```python
from build123d import *

# Parameters (mm, degrees)
SKETCH_R     = 8
SKETCH_W     = 8.42
SKETCH_H     = 2.25
PAD_DEPTH    = 1
SKETCH001_R  = 7
SKETCH001_W  = 8.42
SKETCH001_H  = 2.25
PAD001_DEPTH = 7
SKETCH002_R  = 7
SKETCH002_W  = 7.5
SKETCH002_H  = 1.5
PAD002_DEPTH = 1


with BuildPart() as part:
    # Sketch → Pad (new body)
    with BuildSketch(Plane.XY):
        Circle(SKETCH_R)
        Rectangle(SKETCH_W, SKETCH_H, mode=Mode.SUBTRACT)
    extrude(amount=PAD_DEPTH)

    # Sketch001 (on Face6 of Pad) → Pad001 (join)
    with BuildSketch(Plane(origin=(0, 0, 0), x_dir=(1, 0, 0), z_dir=(0, 0, -1))):
        Circle(SKETCH001_R)
        Rectangle(SKETCH001_W, SKETCH001_H, mode=Mode.SUBTRACT)
    extrude(amount=PAD001_DEPTH)

    # Sketch002 (on Face9 of Pad001) → Pad002 (join)
    with BuildSketch(Plane(origin=(0, 0, -7), x_dir=(1, 0, 0), z_dir=(0, 0, -1))):
        Circle(SKETCH002_R)
        Rectangle(SKETCH002_W, SKETCH002_H, mode=Mode.SUBTRACT)
    extrude(amount=PAD002_DEPTH)


solid = part.part
```
Can you work these out from the model? Positions are in its coordinate system, mm. A direction names the side the tool comes from. Coordinates: 2 decimals unless noted, no trailing zeros. Loops run counter-clockwise (first coordinate to the right, second up) from the corner with the lowest first, then second, coordinate; pieces in that order, holes last. Notation, with made-up numbers: (-9, 61.5) -> (12, 61.5) arc R20 cw to (12, 81.5) -> close; hole circle Ø9 at (71, 84). An arc over 180 degrees is marked (long way). Answer as a JSON object with one key per item and string values.
1) Imagine slicing it at C-C (x = 0). Please give me the cut outline in (y, z) (3 decimals).
Results:
{"outline": "(-8, 0) -> (-7, 0) -> (-7, -8) -> (-0.75, -8) -> (-0.75, -7) -> (-1.125, -7) -> (-1.125, 1) -> (-8, 1) -> close; (0.75, -8) -> (7, -8) -> (7, 0) -> (8, 0) -> (8, 1) -> (1.125, 1) -> (1.125, -7) -> (0.75, -7) -> close"}
2) Imagine slicing it at B-B (z = -5). Please give me the cut outline in (x, y) (3 decimals).
Results:
{"outline": "circle Ø14 at (0, 0); hole (-4.21, -1.125) -> (4.21, -1.125) -> (4.21, 1.125) -> (-4.21, 1.125) -> close"}
3) If I drill on line 1 (Y direction, x = 0, z = -4.5) (3 decimals); line 2 (Y direction, x = -3.5, z = 0.5) (3 decimals); line 3 (Z direction, x = -0.5, y = 7.25), over which ranges is the centre line in solid material (lowest first)?
Results:
{"line 1": "y = -7 to -1.125, 1.125 to 7", "line 2": "y = -7.194 to -1.125, 1.125 to 7.194", "line 3": "z = 0 to 1"}
4) Imagine slicing it at D-D (y = -4). Please give me the cut outline in (x, z), then the cut area to 3 significant figures.
Results:
{"outline": "(-6.93, 0) -> (-5.74, 0) -> (-5.74, -8) -> (5.74, -8) -> (5.74, 0) -> (6.93, 0) -> (6.93, 1) -> (-6.93, 1) -> close", "area": "106 mm^2"}
5) Thinking about a two-plate mould opening in Y: for faces 1 (the face through (-1.73, -7.81, 0.49)), 2 (the face through (3.75, 0, -7.5)), 3 (the face through (0, -2, 1)), which applies, pulls with the +Y half, pulls with the -Y half, needs draft (parallel to the pull), parting line crosses it, or undercut?
Results:
{"face 1": "parting line crosses it", "face 2": "undercut", "face 3": "needs draft"}
6) Imagine slicing it at A-A (y = 0). Please give me the cut outline in (x, z).
Results:
{"outline": "(-8, 0) -> (-7, 0) -> (-7, -8) -> (-3.75, -8) -> (-3.75, -7) -> (-4.21, -7) -> (-4.21, 1) -> (-8, 1) -> close; (3.75, -8) -> (7, -8) -> (7, 0) -> (8, 0) -> (8, 1) -> (4.21, 1) -> (4.21, -7) -> (3.75, -7) -> close"}
7) For P1, Ø2, axis at y = 4.5, z = -2.5, coming from the +X side; P2, Ø3, axis at x = 5, z = -2, coming from the +Y side; P3, Ø1.1, axis at y = 0, z = -7.5, coming from the -X side; P4, Ø4, axis at x = -0.5, z = -1.5, coming from the +Y side, each with a flat end and sliding along its axis, tell me the tip position at first contact or that it passes through.
Results:
{"P1": "stops at x = 6.06", "P2": "stops at y = 6.06", "P3": "stops at x = -7", "P4": "stops at y = 8"}
8) For faces 4 (the face through (-3.75, 0, -7.5)), 5 (the face through (0, 1, -8)), 6 (the face through (4, -6, 0)), 7 (the face through (0, 1.125, -3)), which set-ups out of +Z, -Z, +X, -X, +Y, -Y let a thin tool reach every point of the face, with its end or its side?
Results:
{"face 4": "+Z, -Z", "face 5": "-Z, +X, -X, +Y, -Y", "face 6": "-Z", "face 7": "+Z"}
